from build123d import *

# Parameters (mm, degrees)
F0_R     = 6
F0_R_2   = 6.5
F1_DEPTH = 5
F2_R     = 11.25
F3_DEPTH = 4.1
F5_DEPTH = 4.5


with BuildPart() as f1:
    # F0 (on Top) → F1 (new body, symmetric)
    with BuildSketch(Plane.XY):
        with BuildLine():
            ThreePointArc((12.990381, 18.480762), (14.488887, 22.098476), (15, 25.980762))
            ThreePointArc((15, 25.980762), (-3.882286, 40.46965), (-12.990381, 18.480762))
            ThreePointArc((-12.990381, 18.480762), (0, 10.980762), (12.990381, 18.480762))
        make_face()
        with Locations((0, 25.980762)):
            Circle(F0_R, mode=Mode.SUBTRACT)
        with BuildLine():
            ThreePointArc((12.990381, 18.480762), (0, 10.980762), (-12.990381, 18.480762))
            ThreePointArc((-12.990381, 18.480762), (-12.990381, 7.5), (-22.5, 2.009619))
            ThreePointArc((-22.5, 2.009619), (-11.893398, -2.383779), (-7.5, -12.990381))
            ThreePointArc((-7.5, -12.990381), (-8.011113, -16.872667), (-9.509619, -20.490381))
            ThreePointArc((-9.509619, -20.490381), (0, -15), (9.509619, -20.490381))
            ThreePointArc((9.509619, -20.490381), (9.509619, -5.490381), (22.5, 2.009619))
            ThreePointArc((22.5, 2.009619), (12.990381, 7.5), (12.990381, 18.480762))
        make_face()
        Circle(F0_R_2, mode=Mode.SUBTRACT)
        with BuildLine():
            ThreePointArc((-7.5, -12.990381), (-11.893398, -2.383779), (-22.5, 2.009619))
            ThreePointArc((-22.5, 2.009619), (-35.490381, -20.490381), (-9.509619, -20.490381))
            ThreePointArc((-9.509619, -20.490381), (-8.011113, -16.872667), (-7.5, -12.990381))
        make_face()
        with Locations((-22.5, -12.990381)):
            Circle(F0_R, mode=Mode.SUBTRACT)
        with BuildLine():
            ThreePointArc((37.5, -12.990381), (33.106602, -2.383779), (22.5, 2.009619))
            ThreePointArc((22.5, 2.009619), (9.509619, -5.490381), (9.509619, -20.490381))
            ThreePointArc((9.509619, -20.490381), (26.382286, -27.479268), (37.5, -12.990381))
        make_face()
        with Locations((22.5, -12.990381)):
            Circle(F0_R, mode=Mode.SUBTRACT)
    extrude(amount=F1_DEPTH, both=True)

    # F2 (on Top) → F3 (cut, symmetric)
    with BuildSketch(Plane.XY):
        Circle(F2_R)
    extrude(amount=F3_DEPTH, both=True, mode=Mode.SUBTRACT)

    # F4 (on Top) → F5 (cut, symmetric)
    with BuildSketch(Plane.XY):
        Polygon((27.551815, -4.240381), (17.448185, -4.240381), (12.39637, -12.990381), (17.448185, -21.740381), (27.551815, -21.740381), (32.60363, -12.990381), align=None)
        Polygon((-12.39637, -12.990381), (-17.448185, -4.240381), (-27.551815, -4.240381), (-32.60363, -12.990381), (-27.551815, -21.740381), (-17.448185, -21.740381), align=None)
        Polygon((-5.051815, 17.230762), (5.051815, 17.230762), (10.10363, 25.980762), (5.051815, 34.730762), (-5.051815, 34.730762), (-10.10363, 25.980762), align=None)
    extrude(amount=F5_DEPTH, both=True, mode=Mode.SUBTRACT)


solid = f1.part
Geometry check sheet. Reference: the model listing, model coordinates, mm. A direction names the side the tool comes from. Coordinates: 2 decimals unless noted, no trailing zeros. Order: outer loops, then holes, each group sorted by start corner. A loop starts at its lowest first (then second) coordinate and runs counter-clockwise, first axis right, second up. Notation, with made-up numbers: M 18.25,56 L 58.25,56 A22 cw 58.25,87 Z; hole C 32,-24.75 d7. An arc over 180 degrees is marked long. Use CSV: the item, a comma, the result in double quotes.
Item 1: Mould release check, pull along Y, two halves, no side actions. Record for faces 1 (the flat face through (-20, -7, 4.5)), 2 (the cylindrical face through (0, -15, 0)), 3 (the flat face through (2, 32, -4.5)): pulls with the +Y half, pulls with the -Y half, needs draft (parallel to the pull), parting line crosses it, or undercut.
Returned:
face 1,"undercut"
face 2,"pulls with the -Y half"
face 3,"undercut"
Item 2: Tool access check on faces 4 (the cylindrical face through (-5.158, -3.955, -4.556)), 5 (the flat face through (-14.887, -8.677, -0.063)). Record the directions out of +Z, -Z, +X, -X, +Y, -Y that give a thin tool (end or side, any length) a straight path to the whole face; none if there is none.
Returned:
face 4,"+Z, -Z"
face 5,"none"
Item 3: Cross-section at A-A on x = 0. Record the cut outline in (y, z), then the cut area to 3 significant figures.
Returned:
outline,"M -15,-5 L -6.5,-5 L -6.5,-4.1 L -11.25,-4.1 L -11.25,4.1 L -6.5,4.1 L -6.5,5 L -15,5 Z; M 6.5,-5 L 19.98,-5 L 19.98,-4.5 L 17.23,-4.5 L 17.23,4.5 L 19.98,4.5 L 19.98,5 L 6.5,5 L 6.5,4.1 L 11.25,4.1 L 11.25,-4.1 L 6.5,-4.1 Z; M 31.98,-5 L 40.98,-5 L 40.98,5 L 31.98,5 L 31.98,4.5 L 34.73,4.5 L 34.73,-4.5 L 31.98,-4.5 Z"
area,"182 mm2"
Item 4: Cross-section at D-D on y = -10. Give the number of separate pieces and of enclosed holes in the cut face, then the cut area to 3 significant figures.
Returned:
separate pieces,"3"
enclosed holes,"1"
area,"337 mm2"
Item 5: Cross-section at B-B on y = 0. Record the cut outline in (x, z), then the cut area to 3 significant figures.
Returned:
outline,"M -30,-5 L -6.5,-5 L -6.5,-4.1 L -11.25,-4.1 L -11.25,4.1 L -6.5,4.1 L -6.5,5 L -30,5 Z; M 6.5,-5 L 30,-5 L 30,5 L 6.5,5 L 6.5,4.1 L 11.25,4.1 L 11.25,-4.1 L 6.5,-4.1 Z"
area,"392 mm2"
Item 6: Thickness scan on line 1 along Y through (x, z) = (0, -4.3); line 2 along Y through (x, z) = (-22.5, -4.65); line 3 along Z through (x, y) = (-21.5, -20). Record the ranges inside material, lowest first.
Returned:
line 1,"y = -15 to -6.5, 6.5 to 17.23, 34.73 to 40.98"
line 2,"y = -27.99 to -18.99, -6.99 to 2.01"
line 3,"z = -5 to -4.5, 4.5 to 5"
Item 7: Cross-section at C-C on z = -0.25. Record the cut outline in (x, y).
Returned:
outline,"M -22.5,2.01 A15 ccw long -9.51,-20.49 A10.98 cw 9.51,-20.49 A15 ccw 37.5,-12.99 A15 ccw 22.5,2.01 A10.98 cw 12.99,18.48 A15 ccw 15,25.98 A15 ccw long -12.99,18.48 A10.98 cw Z; hole M -32.6,-12.99 L -27.55,-21.74 L -17.45,-21.74 L -12.4,-12.99 L -17.45,-4.24 L -27.55,-4.24 Z; hole C 0,0 d22.5; hole M -10.1,25.98 L -5.05,17.23 L 5.05,17.23 L 10.1,25.98 L 5.05,34.73 L -5.05,34.73 Z; hole M 12.4,-12.99 L 17.45,-21.74 L 27.55,-21.74 L 32.6,-12.99 L 27.55,-4.24 L 17.45,-4.24 Z"
Item 8: Gauge pin test, flat ends, axial feed: pin 1 Ø5 at (x, z) = (-3, 2.5) entering from -Y; pin 2 Ø1.5 at (x, z) = (-24.5, -3.5) entering from -Y; pin 3 Ø3 at (y, z) = (14.5, 0) entering from +X. Record the tip position at first contact, or that the pin passes through.
Returned:
pin 1,"stops at y = -16.48"
pin 2,"stops at y = -27.94"
pin 3,"stops at x = 11.94"
